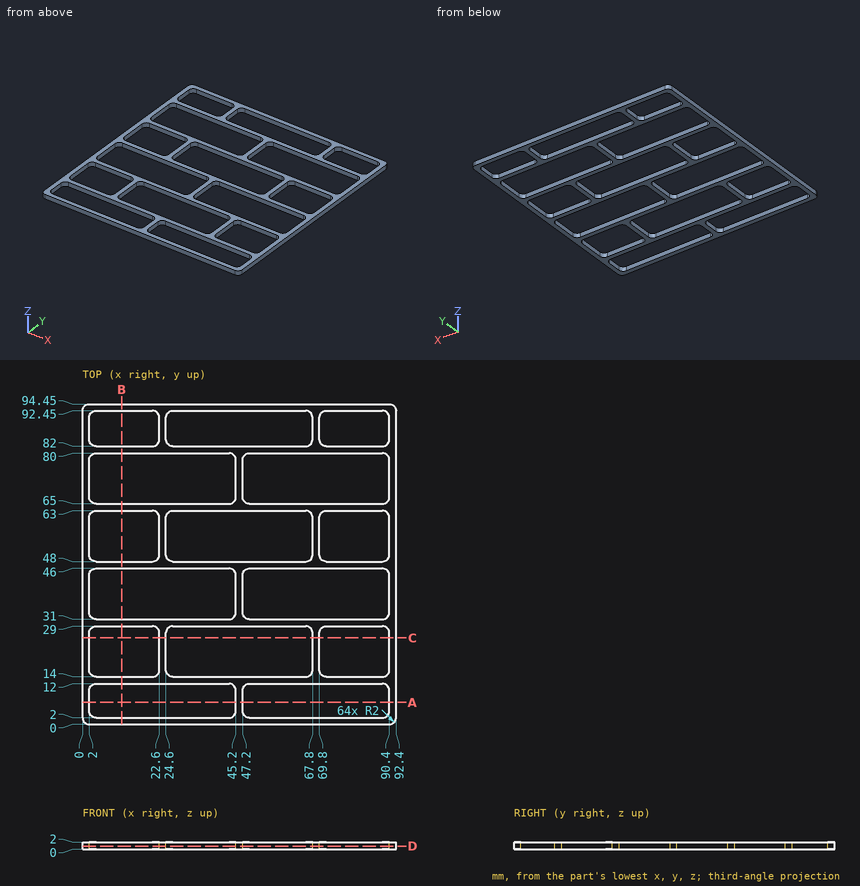
Job drawing, mm, ordinate dimensions from the low corner. One solid piece. Round coordinates to 2 decimals unless told otherwise and drop trailing zeros. Loops run counter-clockwise (first coordinate to the right, second up) from the corner with the lowest first, then second, coordinate; pieces in that order, holes last. Notation, with made-up numbers: (12, -5) -> (69, -5) arc R19 cw to (69, 26) -> close; hole circle Ø1 at (15.5, 60). An arc over 180 degrees is marked (long way). Use CSV: the item, a comma, the result in double quotes. Start each with the question number.
Q1. Saw through at D-D on z = 0.9. Count the separate pieces of the cut face and the enclosed holes in it, and give its area (3 significant figures).
Q2. Flat gauge pin, fed straight in: pin 1 Ø8 at (x, y) = (31, 26.5) entering from +Z. Where does the tip first touch, or does it go through?
Q3. Saw through at C-C on y = 25.5. Give the cut face in (x, z).
Q4. Saw through at A-A on y = 6.5. Give the cut face in (x, z), and give its area (3 significant figures).
Q5. Drill centre lines: L1, parallel to X at y = 41, z = 0.75; L2, parallel to X at y = 23, z = 1.6; L3, parallel to X at y = 49.5, z = 0.3. Where is each one in solid material? Low to high.
Q6. Saw through at B-B on x = 11.5. Give the cut face in (y, z), and give its area (3 significant figures).
Solutions:
1,separate pieces,"1"
1,enclosed holes,"15"
1,area,"1,910 mm^2"
2,pin 1,"stops at z = 2"
3,outline,"(0, 0) -> (2, 0) -> (2, 2) -> (0, 2) -> close; (22.6, 0) -> (24.6, 0) -> (24.6, 2) -> (22.6, 2) -> close; (67.8, 0) -> (69.8, 0) -> (69.8, 2) -> (67.8, 2) -> close; (90.4, 0) -> (92.4, 0) -> (92.4, 2) -> (90.4, 2) -> close"
4,outline,"(0, 0) -> (2, 0) -> (2, 2) -> (0, 2) -> close; (45.2, 0) -> (47.2, 0) -> (47.2, 2) -> (45.2, 2) -> close; (90.4, 0) -> (92.4, 0) -> (92.4, 2) -> (90.4, 2) -> close"
4,area,"12.0 mm^2"
5,L1,"x = 0 to 2, 45.2 to 47.2, 90.4 to 92.4"
5,L2,"x = 0 to 2, 22.6 to 24.6, 67.8 to 69.8, 90.4 to 92.4"
5,L3,"x = 0 to 2.06, 22.54 to 24.66, 67.74 to 69.86, 90.34 to 92.4"
6,outline,"(0, 0) -> (2, 0) -> (2, 2) -> (0, 2) -> close; (12, 0) -> (14, 0) -> (14, 2) -> (12, 2) -> close; (29, 0) -> (31, 0) -> (31, 2) -> (29, 2) -> close; (46, 0) -> (48, 0) -> (48, 2) -> (46, 2) -> close; (63, 0) -> (65, 0) -> (65, 2) -> (63, 2) -> close; (80, 0) -> (82, 0) -> (82, 2) -> (80, 2) -> close; (92.45, 0) -> (94.45, 0) -> (94.45, 2) -> (92.45, 2) -> close"
6,area,"28.0 mm^2"
